Check sheet for the drawn part. Datum: minimum x, y, z corner. Units: mm. A direction names the side the tool comes from. Give positions to 0.01 mm unless a question says otherwise; leave off trailing zeros. Loops run counter-clockwise (first coordinate to the right, second up) from the corner with the lowest first, then second, coordinate; pieces in that order, holes last. Notation, with made-up numbers: (58.5, 33.5) - (95.5, 33.5) arc R14 ccw to (95.5, 57.5) - close; hole circle Ø7 at (20, -39). An arc over 180 degrees is marked (long way). Use one line per item in the form item = value.
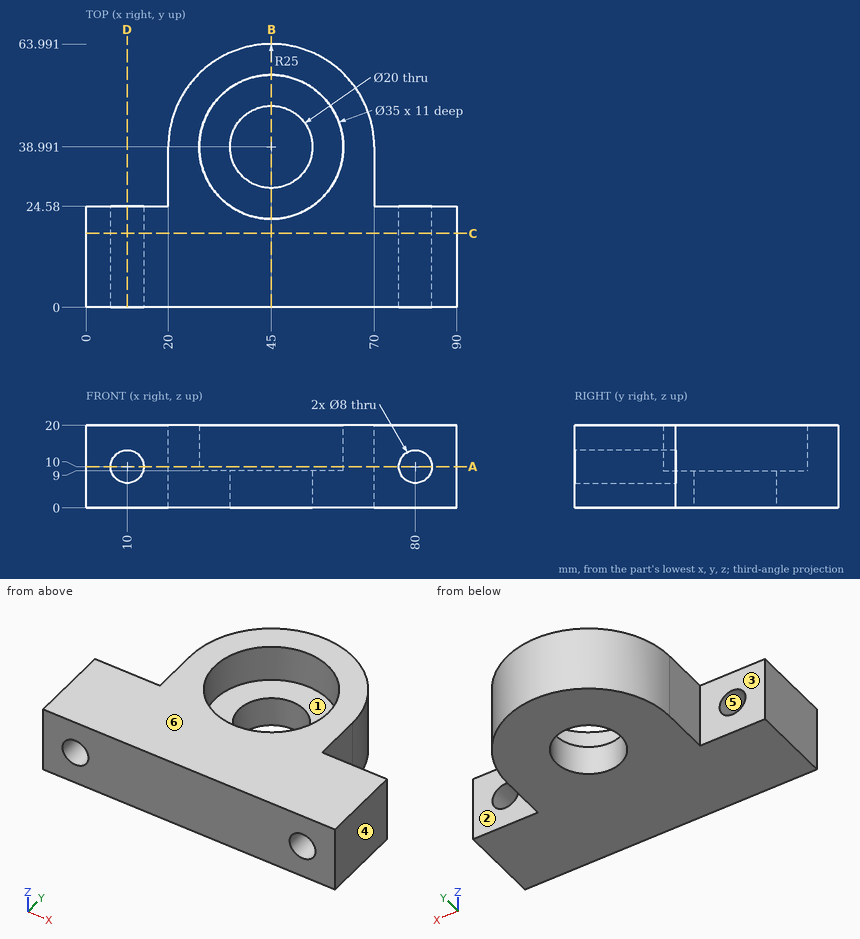
Item 1: Section check D-D on x = 10. Record the boundary of the cut face in (y, z).
Answer block:
outline = (0, 0) - (24.58, 0) - (24.58, 6) - (0, 6) - close; (0, 14) - (24.58, 14) - (24.58, 20) - (0, 20) - close
Item 2: Section check C-C on y = 18. Record the boundary of the cut face in (x, z).
Answer block:
outline = (0, 0) - (90, 0) - (90, 20) - (0, 20) - close; hole circle Ø8 at (10, 10); hole circle Ø8 at (80, 10)
Item 3: Gauge pin test, flat ends, axial feed: P1, Ø8, axis at y = 44, z = 4, coming from the +X side; P2, Ø11.5, axis at y = 33.5, z = 6.5, coming from the -X side; P3, Ø2, axis at x = 33, z = 5.5, coming from the +Y side; P4, Ø5, axis at x = 80, z = 10, coming from the +Y side. Record the tip position at first contact, or that the pin passes through.
Answer block:
P1 = 69.98
P2 = 20
P3 = 61.44
P4 = through
Item 4: Section check B-B on x = 45. Record the boundary of the cut face in (y, z), then the cut area to 3 significant figures.
Answer block:
outline = (0, 0) - (28.99, 0) - (28.99, 9) - (21.49, 9) - (21.49, 20) - (0, 20) - close; (48.99, 0) - (63.99, 0) - (63.99, 20) - (56.49, 20) - (56.49, 9) - (48.99, 9) - close
area = 715 mm2
Item 5: Thickness scan on L1, parallel to X at y = 14, z = 10; L2, parallel to Y at x = 45, z = 3.75; L3, parallel to Y at x = 72.5, z = 2. Record the ranges inside material, lowest first.
Answer block:
L1 = 0 to 6, 14 to 76, 84 to 90
L2 = 0 to 28.99, 48.99 to 63.99
L3 = 0 to 24.58
Item 6: Mould release check, pull along Z, two halves, no side actions. Record for the marked faces 4, 5 and 6: released by +Z, released by -Z, zero draft, split by the parting line, or undercut.
Answer block:
face_4 = zero draft
face_5 = undercut
face_6 = released by +Z
Item 7: Section check A-A on z = 10. Record the boundary of the cut face in (x, y), then the cut area to 3 significant figures.
Answer block:
outline = (0, 0) - (6, 0) - (6, 24.58) - (0, 24.58) - close; (14, 0) - (76, 0) - (76, 24.58) - (70, 24.58) - (70, 38.99) arc R25 ccw to (20, 38.99) - (20, 24.58) - (14, 24.58) - close; (84, 0) - (90, 0) - (90, 24.58) - (84, 24.58) - close; hole circle Ø35 at (45, 38.99)
area = 2,560 mm2
Item 8: Access from +Z, -Z, +X, -X, +Y, -Y to the whole of each face (thin tool, end or side, straight path). Record for the marked faces 1, 2 and 3.
Answer block:
face_1 = +Z
face_2 = +Z, -Z, +X, +Y
face_3 = +Z, -Z, -X, +Y
